from build123d import *

# Parameters (mm, degrees)
F0_W     = 38.1
F0_H     = 101.6
F0_R     = 3.175
F1_DEPTH = 6.35
F2_W     = 10.16
F2_H     = 101.6
F3_DEPTH = 25.4
F4_R     = 6.35
F5_DEPTH = 25.4


with BuildPart() as f1:
    # F0 (on Top) → F1 (new body)
    with BuildSketch(Plane.XY):
        with Locations((19.05, 50.8)):
            Rectangle(F0_W, F0_H)
        with Locations((19.05, 31.75)):
            Circle(F0_R, mode=Mode.SUBTRACT)
        with Locations((19.05, 69.85)):
            Circle(F0_R, mode=Mode.SUBTRACT)
    extrude(amount=F1_DEPTH)

    # F2 (on face) → F3 (join)
    with BuildSketch(Plane.XY.offset(6.35)):
        with Locations((5.08, 50.8)):
            Rectangle(F2_W, F2_H)
    extrude(amount=F3_DEPTH)

    # F4 (on face) → F5 (cut)
    with BuildSketch(Plane(origin=(0, 0, 0), x_dir=(0, -1, 0), z_dir=(-1, 0, 0))):
        with Locations((-82.55, 19.160531)):
            Circle(F4_R)
        with Locations((-57.15, 19.160531)):
            Circle(F4_R)
        Polygon((-31.75, 19.160531), (-31.75, 15.985531), (-12.7, 15.985531), (-12.7, 19.160531), (-12.7, 22.335531), (-31.75, 22.335531), align=None)
    extrude(amount=-F5_DEPTH, mode=Mode.SUBTRACT)


solid = f1.part
Geometry: final body of the model. Coordinates: model frame, mm. A direction names the side the tool comes from. Coordinates: 2 decimals unless noted, no trailing zeros. Order: outer loops, then holes, each group sorted by start corner. A loop starts at its lowest first (then second) coordinate and runs counter-clockwise, first axis right, second up. Notation, with made-up numbers: (-14, 30) - (14, 30) arc R33 cw to (14, 61) - close; hole circle Ø2 at (-9, 27.5). An arc over 180 degrees is marked (long way). Use one line per item in the form item = value.
1) Mould query, pull axis Y, two halves, no side actions, for faces 4 (the face through (18.36, 66.75, 3.13)), 5 (the face through (24, 52, 6.35)), 6 (the face through (10, 101.6, 5)). Classes: +Y half, -Y half, draft (parallel to the pull), parting line (faces both ways), or undercut.
Solutions:
face_4 = undercut
face_5 = draft
face_6 = +Y half
2) Section C-C (z = 24.5). Return loops of the section in (x, y).
Solutions:
outline = (0, 0) - (10.16, 0) - (10.16, 53.71) - (0, 53.71) - close; (0, 60.59) - (10.16, 60.59) - (10.16, 79.11) - (0, 79.11) - close; (0, 85.99) - (10.16, 85.99) - (10.16, 101.6) - (0, 101.6) - close
3) Pin query (flat end, axial travel): pin 1 (2 mm diameter, centred on x = 31, y = 52, fed in from +Z); pin 2 (14.5 mm diameter, centred on y = 57.15, z = 19.16, fed in from +X). Return the tip coordinate at first contact, or that it passes through.
Solutions:
pin_1 = 6.35
pin_2 = 10.16
4) Section A-A (y = 69.85). Return loops of the section in (x, z) (3 decimals).
Solutions:
outline = (0, 0) - (15.875, 0) - (15.875, 6.35) - (10.16, 6.35) - (10.16, 31.75) - (0, 31.75) - close; (22.225, 0) - (38.1, 0) - (38.1, 6.35) - (22.225, 6.35) - close
5) Section B-B (x = 19.05). Return loops of the section in (y, z) (3 decimals).
Solutions:
outline = (0, 0) - (28.575, 0) - (28.575, 6.35) - (0, 6.35) - close; (34.925, 0) - (66.675, 0) - (66.675, 6.35) - (34.925, 6.35) - close; (73.025, 0) - (101.6, 0) - (101.6, 6.35) - (73.025, 6.35) - close
6) Ray query, L1, parallel to Z at x = 8.5, y = 22.5; L2, parallel to Y at x = 8.5, z = 21; L3, parallel to X at y = 38.5, z = 18.5. Return the intervals inside material, ascending.
Solutions:
L1 = 0 to 15.99, 22.34 to 31.75
L2 = 0 to 12.7, 31.75 to 51.07, 63.23 to 76.47, 88.63 to 101.6
L3 = 0 to 10.16
7) Section D-D (y = 82.55). Return loops of the section in (x, z), then the cut area to 3 significant figures.
Solutions:
outline = (0, 0) - (38.1, 0) - (38.1, 6.35) - (10.16, 6.35) - (10.16, 12.81) - (0, 12.81) - close; (0, 25.51) - (10.16, 25.51) - (10.16, 31.75) - (0, 31.75) - close
area = 371 mm^2
8) Set-up query: faces 1 (the face through (5, 22, 15.986)), 2 (the face through (10.16, 50, 19)), 3 (the face through (19, 52, 0)). Return all of +Z, -Z, +X, -X, +Y, -Y with unobstructed straight access to the full face (end or side cutting, diameter ignored); none if empty.
Solutions:
face_1 = +X, -X
face_2 = +Z, +X, +Y, -Y
face_3 = -Z, +X, -X, +Y, -Y
